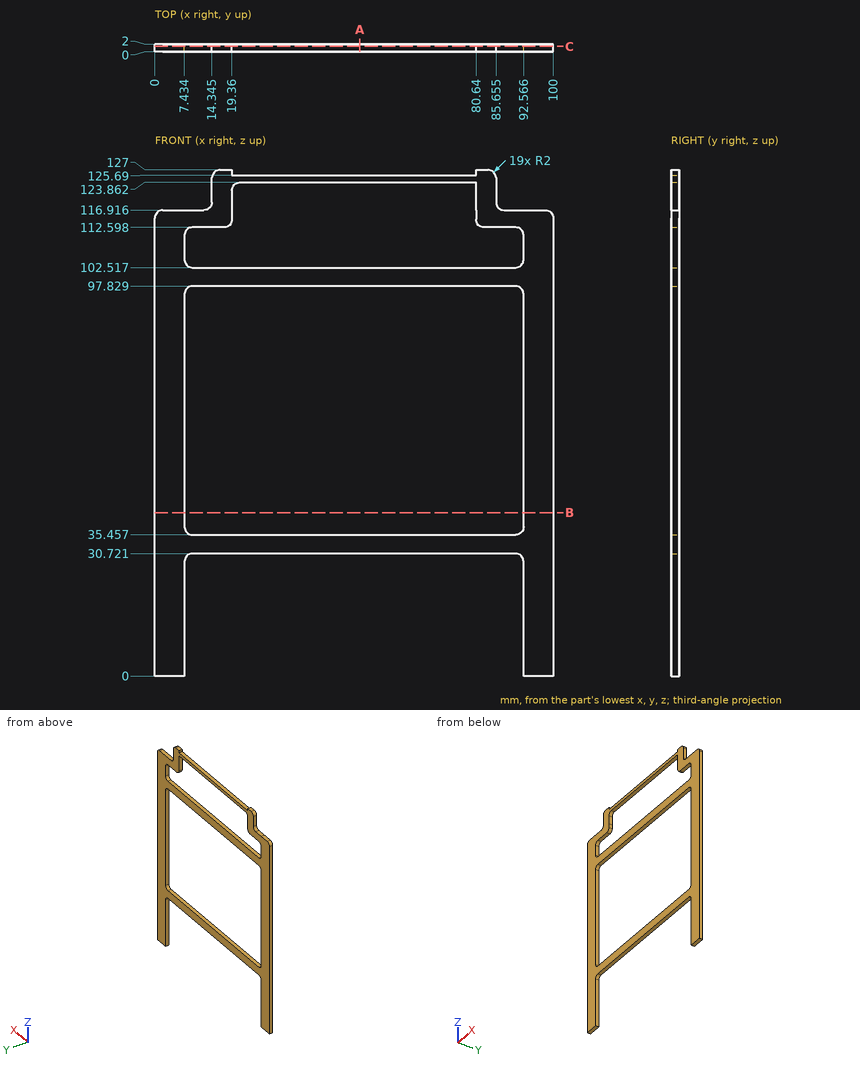
Geometry: see drawing. Coordinates: mm, zero at the bounding-box minimum. Round coordinates to 2 decimals unless told otherwise and drop trailing zeros. Order: outer loops, then holes, each group sorted by start corner. A loop starts at its lowest first (then second) coordinate and runs counter-clockwise, first axis right, second up. Notation, with made-up numbers: (-18, 15) - (34, 15) arc R13 cw to (34, 36) - close; hole circle Ø6 at (17, 40). An arc over 180 degrees is marked (long way). One line per question, with ' | ' between items. Start each with the question number.
1) Cut plane B-B, the plane z = 41. Return the cut outline in (x, y).
2) Cut plane A-A, the plane x = 51.5. Return the cut outline in (y, z), then the cut area to 3 significant figures.
3) Contact query for flat-ended pins moving along their axis: P1, Ø3, axis at x = 89.5, z = 71.5, coming from the +Y side; P2, Ø1, axis at y = 1.5, z = 126.5, coming from the -X side; P3, Ø0.6, axis at x = 93.5, y = 1, coming from the +Z side. Output: stop coordinate, or through.
4) Cut plane C-C, the plane y = 1.4. Give the number of separate pieces and of enclosed holes in the cut face, then the cut area to 3 significant figures.
5) Ray query, probe 1 along Z at (x, y) = (80.5, 1.7); probe 2 along Z at (x, y) = (16, 0.7); probe 3 along X at (y, z) = (1.3, 79). Return the intervals inside material, ascending.
Worked out:
1) outline: (0, 0) - (7.43, 0) - (7.43, 2) - (0, 2) - close; (92.57, 0) - (100, 0) - (100, 2) - (92.57, 2) - close
2) outline: (0, 30.72) - (2, 30.72) - (2, 35.46) - (0, 35.46) - close; (0, 97.83) - (2, 97.83) - (2, 102.52) - (0, 102.52) - close; (0, 123.86) - (2, 123.86) - (2, 125.69) - (0, 125.69) - close | area: 22.5 mm^2
3) P1: passes through | P2: stops at x = 14.61 | P3: stops at z = 116.92
4) separate pieces: 1 | enclosed holes: 2 | area: 2,860 mm^2
5) probe 1: z = 30.72 to 35.46, 97.83 to 102.52, 123.86 to 125.69 | probe 2: z = 30.72 to 35.46, 97.83 to 102.52, 112.6 to 126.97 | probe 3: x = 0 to 7.43, 92.57 to 100
